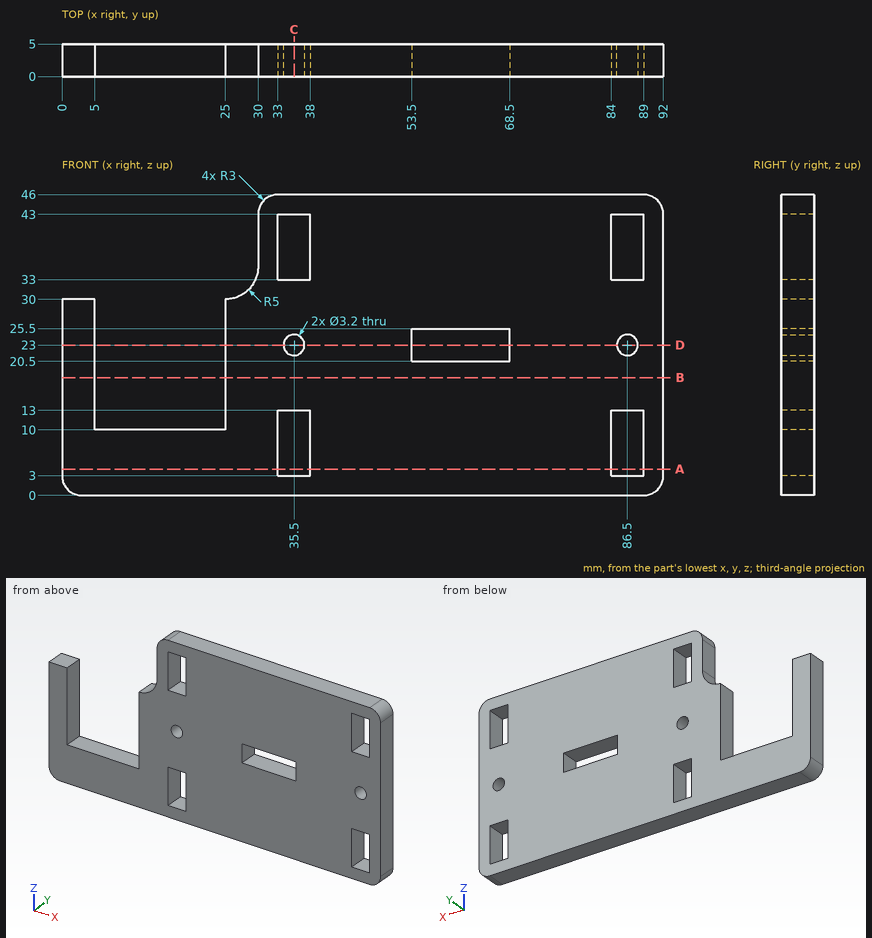
For this review, use the dimensioned drawing (mm, ordinates from the lowest corner) and the shaded views. Give positions to 0.01 mm unless a question says otherwise; leave off trailing zeros. Order: outer loops, then holes, each group sorted by start corner. A loop starts at its lowest first (then second) coordinate and runs counter-clockwise, first axis right, second up. Notation, with made-up numbers: (66.5, 6.5) - (124.5, 6.5) arc R17 cw to (124.5, 30.5) - close; hole circle Ø4 at (9, -29). An arc over 180 degrees is marked (long way). Use CSV: the item, a comma, the result in double quotes. Start each with the question number.
Q1. For P1, Ø2.5, axis at x = 3.5, y = 2, coming from the +Z side; P2, Ø2.5, axis at y = 3, z = 9, coming from the -X side, all flat-tipped, find the tip position at first contact; note any pin that passes through.
Q2. Take a section at A-A (z = 4). State the section outline as (x, y) points.
Q3. Take a section at B-B (z = 18). State the section outline as (x, y) points, and give its area (3 significant figures).
Q4. Take a section at D-D (z = 23). State the section outline as (x, y) points, and give its area (3 significant figures).
Q5. Take a section at C-C (x = 35.5). State the section outline as (y, z) points.
Q6. For line 1 (X direction, y = 4.35, z = 6.5); line 2 (X direction, y = 4, z = 27); line 3 (Z direction, x = 35.5, y = 4), list the stretches that pass through material, from the lowest coordinate up.
Calculated:
1,P1,"stops at z = 30"
1,P2,"stops at x = 0"
2,outline,"(0, 0) - (33, 0) - (33, 5) - (0, 5) - close; (38, 0) - (84, 0) - (84, 5) - (38, 5) - close; (89, 0) - (92, 0) - (92, 5) - (89, 5) - close"
3,outline,"(0, 0) - (5, 0) - (5, 5) - (0, 5) - close; (25, 0) - (92, 0) - (92, 5) - (25, 5) - close"
3,area,"360 mm²"
4,outline,"(0, 0) - (5, 0) - (5, 5) - (0, 5) - close; (25, 0) - (33.9, 0) - (33.9, 5) - (25, 5) - close; (37.1, 0) - (53.5, 0) - (53.5, 5) - (37.1, 5) - close; (68.5, 0) - (84.9, 0) - (84.9, 5) - (68.5, 5) - close; (88.1, 0) - (92, 0) - (92, 5) - (88.1, 5) - close"
4,area,"253 mm²"
5,outline,"(0, 0) - (5, 0) - (5, 3) - (0, 3) - close; (0, 13) - (5, 13) - (5, 21.4) - (0, 21.4) - close; (0, 24.6) - (5, 24.6) - (5, 33) - (0, 33) - close; (0, 43) - (5, 43) - (5, 46) - (0, 46) - close"
6,line 1,"x = 0 to 33, 38 to 84, 89 to 92"
6,line 2,"x = 0 to 5, 25 to 92"
6,line 3,"z = 0 to 3, 13 to 21.4, 24.6 to 33, 43 to 46"
